```python
from build123d import *

# Parameters (mm, degrees)
F0_W            = 40
F0_H            = 40
F1_DEPTH        = 200
F3_DEPTH        = 200
F3_COPIES_COUNT = 4
F4_R            = 5
F5_R            = 4.25
F6_DEPTH        = 200


# Not quite as in the source:
# - a pattern or mirror of a feature is missing from the dataset's text; its kind, count and spacing are read off the source's solid


with BuildPart() as f1:
    # F0 (on Right) → F1 (new body)
    with BuildSketch(Plane.YZ):
        Rectangle(F0_W, F0_H)
    extrude(amount=F1_DEPTH)

    # F2 (on face) → F3 (cut, through all)
    with BuildSketch(Plane.YZ.offset(200)):
        Polygon((4.25, 20), (-4.25, 20), (-4.25, 17), (-6.5, 17), (-6.5, 12), (6.5, 12), (6.5, 17), (4.25, 17), align=None)
    f3 = extrude(amount=-F3_DEPTH, mode=Mode.SUBTRACT)

    # F3_copies: F3 ×4 about axis
    f3_copies_axis = Axis((0, 0, 0), (1, 0, 0))
    for i in range(1, F3_COPIES_COUNT):
        add(f3.rotate(f3_copies_axis, i * 360 / F3_COPIES_COUNT), mode=Mode.SUBTRACT)

    # F4
    f4_edges = [f1.edges().sort_by_distance(p)[0] for p in [
        (100, 20, 20),
        (100, -20, 20),
        (100, 20, -20),
        (100, -20, -20),
    ]]
    fillet(f4_edges, radius=F4_R)

    # F5 (on face) → F6 (cut, through all)
    with BuildSketch(Plane.YZ.offset(200)):
        Circle(F5_R)
    extrude(amount=-F6_DEPTH, mode=Mode.SUBTRACT)


solid = f1.part
```
Input: part model. Units: mm. Frame: model coordinates. A direction names the side the tool comes from. Round coordinates to 2 decimals unless told otherwise and drop trailing zeros. Loops run counter-clockwise (first coordinate to the right, second up) from the corner with the lowest first, then second, coordinate; pieces in that order, holes last. Notation, with made-up numbers: M 59.5,-13 L 64.5,-13 A22 ccw 64.5,13 Z; hole C 64.25,59.5 d9. An arc over 180 degrees is marked long. Answer in a Markdown table with one row per item. Add a question column.
1. Ray query, probe 1 along Z at (x, y) = (51, 0); probe 2 along Y at (x, z) = (136, -5); probe 3 along Z at (x, y) = (125.5, 15). Return the intervals inside material, ascending.
2. Mould query, pull axis Y, two halves, no side actions, for faces 3 (the face through (200, -5, 0)), 4 (the face through (101, 18, 19)), 5 (the face through (101, -12, 0)), 6 (the face through (101, -6.5, 15)). Classes: released by +Y, released by -Y, zero draft, split by the parting line, or undercut.
3. Contact query for flat-ended pins moving along their axis: pin 1 (2.5 mm diameter, centred on x = 104.5, y = 18, fed in from -Z); pin 2 (1.5 mm diameter, centred on x = 132, y = -19, fed in from -Z); pin 3 (3 mm diameter, centred on y = -11.5, z = 4.5, fed in from -X). Output: stop coordinate, or through.
4. Set-up query: faces 1 (the face through (99, -10, 20)), 2 (the face through (101, -6.5, -14)). Return all of +Z, -Z, +X, -X, +Y, -Y with unobstructed straight access to the full face (end or side cutting, diameter ignored); none if empty.
5. Section A-A (z = 0). Output: boundary loops of the cut face in (x, y), and give its area (3 significant figures).
Values follow:
| question | item | result |
|---|---|---|
| 1 | probe 1 | -12 to -4.25, 4.25 to 12 |
| 1 | probe 2 | -20 to -17, -12 to 12, 17 to 20 |
| 1 | probe 3 | -20 to -6.5, 6.5 to 20 |
| 2 | face 3 | zero draft |
| 2 | face 4 | released by +Y |
| 2 | face 5 | undercut |
| 2 | face 6 | undercut |
| 3 | pin 1 | z = -19.68 |
| 3 | pin 2 | z = -18.8 |
| 3 | pin 3 | x = 0 |
| 4 | face 1 | +Z, +X, -X, +Y, -Y |
| 4 | face 2 | +X, -X |
| 5 | outline | M 0,-12 L 200,-12 L 200,-4.25 L 0,-4.25 Z; M 0,4.25 L 200,4.25 L 200,12 L 0,12 Z |
| 5 | area | 3,100 mm^2 |
